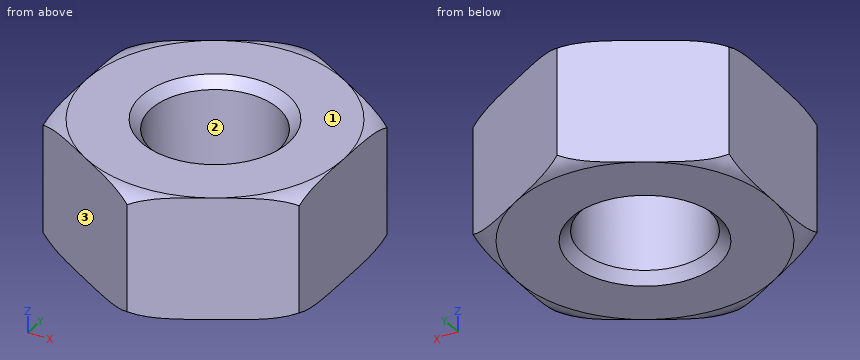
```python
from build123d import *

# Parameters (mm, degrees)
F2_R     = 8.530956
F3_DEPTH = 12.5


with BuildPart() as f1:
    # F0 (on Front) → F1 (revolve)
    with BuildSketch(Plane.XZ):
        with BuildLine():
            Line((-3.25, -2.625), (-3.25, 0))
            Line((-3.25, 0), (-3.25, 2.625))
            Line((-3.25, 2.625), (-3.75, 3.125))
            Line((-3.75, 3.125), (-6.5, 3.125))
            ThreePointArc((-6.5, 3.125), (-7.036601, 3.028199), (-7.505553, 2.75))
            Line((-7.505553, 2.75), (-7.505553, 0))
            Line((-7.505553, 0), (-7.505553, -2.75))
            ThreePointArc((-7.505553, -2.75), (-7.036601, -3.028199), (-6.5, -3.125))
            Line((-6.5, -3.125), (-3.75, -3.125))
            Line((-3.75, -3.125), (-3.25, -2.625))
        make_face()
    revolve(axis=Axis((0, 0, 4.430122), (0, 0, 1)))

    # F2 (on Top) → F3 (cut, symmetric)
    with BuildSketch(Plane.XY):
        Circle(F2_R)
        Polygon((0, 7.505553), (6.5, 3.752777), (6.5, -3.752777), (0, -7.505553), (-6.5, -3.752777), (-6.5, 3.752777), align=None, mode=Mode.SUBTRACT)
    extrude(amount=F3_DEPTH, both=True, mode=Mode.SUBTRACT)


solid = f1.part
```
Design review of the part built by this model. Coordinates are the model's own, in mm. Face numbers are marked on the shaded views. Round coordinates to 2 decimals unless told otherwise and drop trailing zeros. Return JSON: item names as keys, results as strings.
Q1. The part is to be moulded in two halves that separate along Y. For the marked faces 1, 2 and 3, say which applies: pulls with the +Y half, pulls with the -Y half, needs draft (parallel to the pull), parting line crosses it, or undercut.
Computed values:
{"face 1": "needs draft", "face 2": "undercut", "face 3": "pulls with the -Y half"}
Q2. For pin 1 Ø1 at (y, z) = (4, -1) entering from -X, flat-tipped, find the tip position at first contact; note if it passes through.
Computed values:
{"pin 1": "stops at x = -6.5"}
Q3. Wall thickness on L1, parallel to X at y = 0, z = -0.4; L2, parallel to Y at x = -1.5, z = 3; L3, parallel to Y at x = 2.5, z = 2.75: over which ranges is each line inside the solid? List them lowest first. Write a range as [from, to].
Computed values:
{"L1": "x = [-6.5, -3.25], [3.25, 6.5]", "L2": "y = [-6.64, -3.3], [3.3, 6.64]", "L3": "y = [-6.06, -2.27], [2.27, 6.06]"}
